Could you check a few things on this model? Use its own coordinates, in mm. A direction names the side the tool comes from. Round coordinates to 2 decimals unless told otherwise and drop trailing zeros. Write each loop counter-clockwise with the first axis right and the second up, starting at its lowest first coordinate (ties: lowest second). Pieces come first, ordered by that corner, then holes. Notation, with made-up numbers: (10.25, -34) -> (31.25, -34) arc R8 ccw to (31.25, -22) -> close; hole circle Ø5 at (-13, 78). An arc over 180 degrees is marked (long way). Answer in a Markdown table with one row per item.
Autodesk Inventor part; units mm, degrees
ref_plane "YZ Plane" through (0, 0, 0) normal (1, 0, 0) x (0, 1, 0)
ref_plane "XZ Plane" through (0, 0, 0) normal (0, 1, 0) x (-1, 0, 0)
ref_plane "XY Plane" through (0, 0, 0) normal (0, 0, 1) x (1, 0, 0)
sketch "Skizze1" plane through (0, 0, 0) normal (0, 1, 0) x (-1, 0, 0)
  arc A0 (4, -6.9282) -> (0, 8) centre (0, 0) ccw
  line L0 (0, -22) -> (0, -27)
  line L1 (0, -27) -> (30, -27)
  line L2 (80, 8) -> (0, 8)
  line L3 (0, -22) -> (25, -22)
  line L4 (25, -22) -> (0, -22)
  line L5 (25, -22) -> (25, -16.2)
  line L6 (25, -16) -> (25, -22)
  line L7 (25, -16.2) -> (16.7663, -16.2)
  line L8 (16.7663, -16.2) -> (4, -6.9282)
  line L9 (30, -27) -> (80, -27)
  line L10 (80, -27) -> (80, -18.6)
  line L11 (80, -18.6) -> (30, -18.6)
  line L12 (80, 1.45) -> (30, 1.45)
  line L13 (30, -18.6) -> (30, 1.45)
  line L14 (80, 1.45) -> (160, 1.45)
  line L15 (80, 1.45) -> (160, 1.45) construction
  line L16 (160, 1.45) -> (160, 26.45)
  line L17 (160, 26.45) -> (105, 26.45)
  line L18 (80, 8) -> (105, 8)
  line L19 (105, 8) -> (105, 26.45)
  circle A1 centre (119.5, 13.95) radius 8.025
  circle A2 centre (145.5, 13.95) radius 8.025
  dimension "d0" = 5
  dimension "d9" = 50
  dimension "d10" = 8.4
  dimension "d12" = 20.05
  dimension "d17" = 0
  dimension "d18" = 25
  dimension "d19" = 55
  dimension "d20" = 160
  dimension "d21" = 8
  dimension "d22" = 30
  dimension "d23" = 16.05
  dimension "d24" = 16.05
  dimension "d25" = 12.5
  dimension "d26" = 12.5
  dimension "d28" = 26
  dimension "d29" = 14.5
extrude "Extrusion1" add sketch "Skizze1" along normal blind 20 contours A0 L2 L18 L19 L17 L16 L14 L12 L13 L11 L10 L9 L1 L0 L3 L5 L7 L8 | A1 | A2
properties part number "Halterung_MobileWhiteboard_V3_Ultrasonic scanner"
1) For faces 5 (the face through (-94, 10, 1.45)), 6 (the face through (-25, 10, -19)), 7 (the face through (-105, 10, 17)), which set-ups out of +Z, -Z, +X, -X, +Y, -Y let a thin tool reach every point of the face, with its end or its side?
Findings:
| item | result |
|---|---|
| face 5 | -X, +Y, -Y |
| face 6 | +X, +Y, -Y |
| face 7 | +Z, +X, +Y, -Y |
2) Imagine slicing it at D-D, the plane z = 14. Please give me the cut outline in (x, y).
Findings:
| item | result |
|---|---|
| outline | (-160, 0) -> (-105, 0) -> (-105, 20) -> (-160, 20) -> close |
3) For pin 1 (2 mm diameter, centred on y = 16, z = -6, fed in from -X); pin 2 (10 mm diameter, centred on x = -51, y = 17.5, fed in from +Z); pin 3 (1.7 mm diameter, centred on y = 13, z = -18.5, fed in from +X), each with a flat end and sliding along its axis, tell me the tip position at first contact or that it passes through.
Findings:
| item | result |
|---|---|
| pin 1 | stops at x = -30 |
| pin 2 | stops at z = 8 |
| pin 3 | stops at x = -25 |
4) Thinking about a two-plate mould opening in Z: for faces 1 (the face through (-7.69, 9.86, 2.21)), 2 (the face through (-80, 10, -23)), 3 (the face through (-21, 10, -16.2)), 4 (the face through (-39, 10, -27)), which applies, +Z half, -Z half, draft (parallel to the pull), parting line (faces both ways), or undercut?
Findings:
| item | result |
|---|---|
| face 1 | undercut |
| face 2 | draft |
| face 3 | undercut |
| face 4 | -Z half |
5) Imagine slicing it at A-A, the plane x = -44. Please give me the cut outline in (y, z), plus the area to 3 significant figures.
Findings:
| item | result |
|---|---|
| outline | (0, -27) -> (20, -27) -> (20, -18.6) -> (0, -18.6) -> close; (0, 1.45) -> (20, 1.45) -> (20, 8) -> (0, 8) -> close |
| area | 299 mm^2 |
6) Please list where these lines run through material, in increasing order: line 1 (Z direction, x = -22, y = 16.75); line 2 (Z direction, x = -74, y = 16); line 3 (Z direction, x = -149.5, y = 6.75).
Findings:
| item | result |
|---|---|
| line 1 | z = -27 to -22, -16.2 to 8 |
| line 2 | z = -27 to -18.6, 1.45 to 8 |
| line 3 | z = 1.45 to 26.45 |
7) Imagine slicing it at C-C, the plane x = -92. Please give me the cut outline in (y, z), plus the area to 3 significant figures.
Findings:
| item | result |
|---|---|
| outline | (0, 1.45) -> (20, 1.45) -> (20, 8) -> (0, 8) -> close |
| area | 131 mm^2 |
8) Imagine slicing it at B-B, the plane y = 16. Please give me the cut outline in (x, z).
Findings:
| item | result |
|---|---|
| outline | (-160, 1.45) -> (-30, 1.45) -> (-30, -18.6) -> (-80, -18.6) -> (-80, -27) -> (0, -27) -> (0, -22) -> (-25, -22) -> (-25, -16.2) -> (-16.77, -16.2) -> (-4, -6.93) arc R8 cw to (0, 8) -> (-105, 8) -> (-105, 26.45) -> (-160, 26.45) -> close |
